Can you work these out from the model? Positions are in its coordinate system, mm. Round coordinates to 2 decimals unless told otherwise and drop trailing zeros. Order: outer loops, then holes, each group sorted by start corner. A loop starts at its lowest first (then second) coordinate and runs counter-clockwise, first axis right, second up. Notation, with made-up numbers: (15, -34.5) -> (61, -34.5) arc R14 ccw to (61, -10.5) -> close; hole circle Ø1 at (73, -31). An arc over 180 degrees is marked (long way). One line per item, written item: value.
```python
from build123d import *

# Parameters (mm, degrees)
SCHIZZO1_R                   = 55
ESTRUSIONE_ESTRUSIONE1_DEPTH = 4
SCHIZZO2_R                   = 8
SCHIZZO2_R_2                 = 1.6
TAGLIO_ESTRUSIONE1_DEPTH     = 78.884529914


with BuildPart() as part:
    # Schizzo1 → Estrusione-Estrusione1 (new body)
    with BuildSketch(Plane(origin=(0, 0, 0), x_dir=(1, 0, 0), z_dir=(0, 1, 0))):
        with Locations(Location((0, 0, 0), (0, 0, 270))):
            Circle(SCHIZZO1_R)
    extrude(amount=ESTRUSIONE_ESTRUSIONE1_DEPTH)

    # Schizzo2 → Taglio-Estrusione1 (cut, through all)
    with BuildSketch(Plane(origin=(0, 4, 0), x_dir=(1, 0, 0), z_dir=(0, 1, 0))):
        with Locations(Location((0, 0, 0), (0, 0, 270))):
            Circle(SCHIZZO2_R)
        with Locations(Location((0, 47, 0), (0, 0, 270))):
            Circle(SCHIZZO2_R_2)
        with Locations(Location((40.703193978, -23.5, 0), (0, 0, 270))):
            Circle(SCHIZZO2_R_2)
        with Locations(Location((-40.703193978, -23.5, 0), (0, 0, 270))):
            Circle(SCHIZZO2_R_2)
    extrude(amount=-TAGLIO_ESTRUSIONE1_DEPTH, mode=Mode.SUBTRACT)


solid = part.part
```
Q1. I want a section at C-C on y = 1.8. List the corners of the cut face in (x, z) for me, plus the area to 3 significant figures.
Answers below:
outline: circle Ø110 at (0, 0); hole circle Ø3.2 at (-40.7, 23.5); hole circle Ø16 at (0, 0); hole circle Ø3.2 at (0, -47); hole circle Ø3.2 at (40.7, 23.5)
area: 9,280 mm^2
Q2. I want a section at D-D on z = -47. List the corners of the cut face in (x, y) for me, plus the area to 3 significant figures.
Answers below:
outline: (-28.57, 0) -> (-1.6, 0) -> (-1.6, 4) -> (-28.57, 4) -> close; (1.6, 0) -> (28.57, 0) -> (28.57, 4) -> (1.6, 4) -> close
area: 216 mm^2
Q3. Will these pins go through, and if not, where does the flat tip stop? pin 1 Ø4 at (x, z) = (-16, 22.5) entering from -Y; pin 2 Ø2 at (y, z) = (2, 33) entering from -X; pin 3 Ø2 at (x, y) = (41.5, 1.5) entering from -Z.
Answers below:
pin 1: y = 0
pin 2: x = -44.73
pin 3: z = -37.21
Q4. Please list where these lines run through material, in increasing order: line 1 along X through (y, z) = (3.2, 23.5); line 2 along X through (y, z) = (3.15, 0); line 3 along X through (y, z) = (0.5, 22.5).
Answers below:
line 1: -49.73 to -42.3, -39.1 to 39.1, 42.3 to 49.73
line 2: -55 to -8, 8 to 55
line 3: -50.19 to -41.95, -39.45 to 39.45, 41.95 to 50.19
Q5. I want a section at A-A on x = 0. List the corners of the cut face in (y, z) for me.
Answers below:
outline: (0, -55) -> (4, -55) -> (4, -48.6) -> (0, -48.6) -> close; (0, -45.4) -> (4, -45.4) -> (4, -8) -> (0, -8) -> close; (0, 8) -> (4, 8) -> (4, 55) -> (0, 55) -> close
Q6. We'd pull the mould along X, two halves only. Please class faces 1 (the face through (-48.794, 1.972, 25.379)), 2 (the face through (-11, 0, -1)), 3 (the face through (0.481, 2.028, -45.474)): released by +X, released by -X, zero draft, split by the parting line, or undercut.
Answers below:
face 1: split by the parting line
face 2: zero draft
face 3: undercut
Q7. I want a section at B-B on z = 0. List the corners of the cut face in (x, y) for me.
Answers below:
outline: (-55, 0) -> (-8, 0) -> (-8, 4) -> (-55, 4) -> close; (8, 0) -> (55, 0) -> (55, 4) -> (8, 4) -> close
